Part model, mm, in its own coordinate system. A direction names the side the tool comes from. Give positions to 0.01 mm unless a question says otherwise; leave off trailing zeros. Order: outer loops, then holes, each group sorted by start corner. A loop starts at its lowest first (then second) coordinate and runs counter-clockwise, first axis right, second up. Notation, with made-up numbers: (52, 16) -> (64, 16) arc R19 cw to (64, 43) -> close; hole circle Ø5 at (80, 71). An arc over 180 degrees is marked (long way). Write item = value, one per line. Start each with the question number.
Item 1: Pull direction Y, two halves, no side cores. Call faces 3 (the face through (139.151, 34.656, -7.696)), 4 (the face through (135.7, 26, 16)), 5 (the face through (141.22, 26.36, -5.85)): +Y half, -Y half, draft (parallel to the pull), parting line (faces both ways), or undercut.
Item 2: Band-saw the part on C-C on z = 0. Write the cut outline in (x, y), plus the area to 3 significant figures.
Item 3: Band-saw the part on B-B on z = -20. Write the cut outline in (x, y).
Item 4: Tool access for faces 1 (the face through (139.15, 16.75, -29.72)), 2 (the face through (139.7, -20.3, -18.1)): list every direction of +Z, -Z, +X, -X, +Y, -Y with a clear straight run to the whole face (end or side of a thin tool).
Item 5: Drill centre lines: line 1 along Y through (x, z) = (140.75, 0); line 2 along Y through (x, z) = (137.65, 0); line 3 along Z through (x, y) = (139, 16.25). Where is each one in solid material? Low to high.
Item 6: Flat gauge pins, fed straight in: P1, Ø4, axis at y = 11.5, z = -22, coming from the +X side; P2, Ø3, axis at x = 139, y = -15, coming from the -Z side; P3, Ø1.5, axis at x = 141.5, z = 5.5, coming from the +Y side; P4, Ø1, axis at x = 141.5, y = 25, coming from the +Z side. Where does each tip first touch, or does it go through?
Item 7: Band-saw the part on A-A on y = 0. Write the cut outline in (x, z), plus the area to 3 significant figures.
Item 8: Band-saw the part on D-D on y = 16.25. Write the cut outline in (x, z).
```python
from build123d import *

# Parameters (mm, degrees)
AXIAL_HOLES_DEPTH      = 152.273890675
AXIAL_HOLES_DEPTH_BACK = 152.273890675
SKETCH2_R              = 1.65


with BuildPart() as part:
    # Axial profile (mm) → Full revolution (revolve)
    with BuildSketch(Plane.XY, mode=Mode.PRIVATE) as full_revolution_sk:
        Polygon((135.7, 30.25), (139.7, 30.25), (139.7, 27), (142.7, 27), (142.7, 35.5), (135.7, 35.5), align=None)
    revolve(full_revolution_sk.sketch.rotate(Axis((-110, 0, 0), (1, 0, 0)), 90), axis=Axis((-110, 0, 0), (1, 0, 0)))

    # Sketch2 → Axial holes (cut, two sides: drawn at the far end of the back side and taken through both)
    with BuildSketch(Plane(origin=(0, 0, 0), x_dir=(0, 0, -1), z_dir=(1, 0, 0)).offset(-AXIAL_HOLES_DEPTH_BACK)):
        with Locations((-28.145825623, 16.25)):
            Circle(SKETCH2_R)
        with Locations((0, -32.5)):
            Circle(SKETCH2_R)
        with Locations((28.145825623, 16.25)):
            Circle(SKETCH2_R)
    extrude(amount=AXIAL_HOLES_DEPTH + AXIAL_HOLES_DEPTH_BACK, mode=Mode.SUBTRACT)


solid = part.part
```
Values found:
q1.face_3 = parting line
q1.face_4 = draft
q1.face_5 = undercut
q2.outline = (135.7, -35.5) -> (142.7, -35.5) -> (142.7, -34.15) -> (135.7, -34.15) -> close; (135.7, -30.85) -> (142.7, -30.85) -> (142.7, -27) -> (139.7, -27) -> (139.7, -30.25) -> (135.7, -30.25) -> close; (135.7, 30.25) -> (139.7, 30.25) -> (139.7, 27) -> (142.7, 27) -> (142.7, 35.5) -> (135.7, 35.5) -> close
q2.area = 69.9 mm^2
q3.outline = (135.7, -29.33) -> (142.7, -29.33) -> (142.7, -18.14) -> (139.7, -18.14) -> (139.7, -22.69) -> (135.7, -22.69) -> close; (135.7, 22.69) -> (139.7, 22.69) -> (139.7, 18.14) -> (142.7, 18.14) -> (142.7, 29.33) -> (135.7, 29.33) -> close
q4.face_1 = +X, -X
q4.face_2 = -X
q5.line_1 = -35.5 to -34.15, -30.85 to -27, 27 to 35.5
q5.line_2 = -35.5 to -34.15, -30.85 to -30.25, 30.25 to 35.5
q5.line_3 = -31.56 to -29.8, -26.5 to -25.51, 25.51 to 26.5, 29.8 to 31.56
q6.P1 = through
q6.P2 = -32.83
q6.P3 = 35.18
q6.P4 = 25.69
q7.outline = (135.7, -35.5) -> (142.7, -35.5) -> (142.7, -27) -> (139.7, -27) -> (139.7, -30.25) -> (135.7, -30.25) -> close; (135.7, 30.25) -> (139.7, 30.25) -> (139.7, 27) -> (142.7, 27) -> (142.7, 35.5) -> (135.7, 35.5) -> close
q7.area = 93.0 mm^2
q8.outline = (135.7, -31.56) -> (142.7, -31.56) -> (142.7, -29.8) -> (135.7, -29.8) -> close; (135.7, -26.5) -> (142.7, -26.5) -> (142.7, -21.56) -> (139.7, -21.56) -> (139.7, -25.51) -> (135.7, -25.51) -> close; (135.7, 25.51) -> (139.7, 25.51) -> (139.7, 21.56) -> (142.7, 21.56) -> (142.7, 26.5) -> (135.7, 26.5) -> close; (135.7, 29.8) -> (142.7, 29.8) -> (142.7, 31.56) -> (135.7, 31.56) -> close
